The listing builds one solid part. Answer for the finished solid, in the listing's coordinates (mm). A direction names the side the tool comes from. Give positions to 0.01 mm unless a question says otherwise; leave off trailing zeros. Write each loop counter-clockwise with the first axis right and the second up, starting at its lowest first coordinate (ties: lowest second). Pieces come first, ordered by that corner, then holes.
```python
from build123d import *

# Parameters (mm, degrees)
SKETCH_1_R      = 1.6
EXTRUDE_1_DEPTH = 2.5
FILLET_1_R      = 2


with BuildPart() as part:
    # 草图1 → 凸台-拉伸1 (new body)
    with BuildSketch(Plane(origin=(0, 0, 0), x_dir=(-1, 0, 0), z_dir=(0, 1, 0))):
        Polygon((-27.5, 21.5), (27.5, 21.5), (33.5, 21.5), (33.5, -12.5), (27.5, -12.5), (27.5, -21.5), (-27.5, -21.5), align=None)
        with Locations(Location((-24.5, 9.5, 0), (0, 0, 90))):
            Circle(SKETCH_1_R, mode=Mode.SUBTRACT)
        with Locations(Location((-9.5, 9.5, 0), (0, 0, 90))):
            Circle(SKETCH_1_R, mode=Mode.SUBTRACT)
        with Locations(Location((-24.5, -6.5, 0), (0, 0, 90))):
            Circle(SKETCH_1_R, mode=Mode.SUBTRACT)
        with Locations(Location((-9.5, -6.5, 0), (0, 0, 90))):
            Circle(SKETCH_1_R, mode=Mode.SUBTRACT)
        with Locations(Location((4.5, -2.5, 0), (0, 0, 90))):
            Circle(SKETCH_1_R, mode=Mode.SUBTRACT)
        with Locations(Location((4.5, 11.5, 0), (0, 0, 90))):
            Circle(SKETCH_1_R, mode=Mode.SUBTRACT)
        with Locations(Location((24.5, 11.5, 0), (0, 0, 90))):
            Circle(SKETCH_1_R, mode=Mode.SUBTRACT)
        with Locations(Location((16.5, -14.5, 0), (0, 0, 90))):
            Circle(SKETCH_1_R, mode=Mode.SUBTRACT)
        with Locations(Location((4.5, -18, 0), (0, 0, 90))):
            Circle(SKETCH_1_R, mode=Mode.SUBTRACT)
    extrude(amount=EXTRUDE_1_DEPTH)

    # 圆角1
    fillet_1_edges = [part.edges().sort_by_distance(p)[0] for p in [
        (27.5, 1.25, 21.5),
        (-33.5, 1.25, 21.5),
        (-33.5, 1.25, -12.5),
        (-27.5, 1.25, -12.5),
        (-27.5, 1.25, -21.5),
        (27.5, 1.25, -21.5),
    ]]
    fillet(fillet_1_edges, radius=FILLET_1_R)


solid = part.part
```
Item 1: A cutting plane is placed at A-A, the plane z = -2.5. Give the vertices of the cut face in (x, y), plus the area to 4 significant figures.
Conclusion:
outline: (-33.5, 0) - (-6.1, 0) - (-6.1, 2.5) - (-33.5, 2.5) - close; (-2.9, 0) - (27.5, 0) - (27.5, 2.5) - (-2.9, 2.5) - close
area: 144.5 mm2
Item 2: A cutting plane is placed at D-D, the plane x = -4.5. Give the vertices of the cut face in (y, z), plus the area to 3 significant figures.
Conclusion:
outline: (0, -21.5) - (2.5, -21.5) - (2.5, -19.6) - (0, -19.6) - close; (0, -16.4) - (2.5, -16.4) - (2.5, -4.1) - (0, -4.1) - close; (0, -0.9) - (2.5, -0.9) - (2.5, 9.9) - (0, 9.9) - close; (0, 13.1) - (2.5, 13.1) - (2.5, 21.5) - (0, 21.5) - close
area: 83.5 mm2
Item 3: This flat-tipped pin is pushed along its axis until it touches: P1, Ø0.6, axis at x = -30.5, y = 1.5, coming from the -Z side. Where does it stop, or does it pass through?
Conclusion:
P1: stops at z = -12.5
Item 4: Which of the six approach directions +Z, -Z, +X, -X, +Y, -Y give full straight-line access (tool end or side, diameter ignored) to faces 1 (the face through (-15.42, 1.23, -15.68)), 2 (the face through (-31, 1, -12.5))?
Conclusion:
face 1: +Y, -Y
face 2: -Z, -X, +Y, -Y
Item 5: A cutting plane is placed at C-C, the plane y = 0.55. Count the separate pieces of the cut face and the enclosed holes in it, plus the area to 3 significant figures.
Conclusion:
separate pieces: 1
enclosed holes: 9
area: 2,490 mm2
Item 6: Determine the mould class of faces 3 (the face through (-3, 2.5, 0)), 4 (the face through (-33.5, 1, 5)), 5 (the face through (-24.43, 1.23, 9.9)), 6 (the face through (27.5, 1, 0)) for opening direction X: pulls with the +X half, pulls with the -X half, needs draft (parallel to the pull), parting line crosses it, or undercut.
Conclusion:
face 3: needs draft
face 4: pulls with the -X half
face 5: undercut
face 6: pulls with the +X half
Item 7: Consider probe 1 along X at (y, z) = (1.3, 11.5); probe 2 along X at (y, z) = (1.2, -6.5); probe 3 along X at (y, z) = (1.45, -14.5). Determine where each line is inside the solid, lowest interval first.
Conclusion:
probe 1: x = -33.5 to -26.1, -22.9 to -6.1, -2.9 to 27.5
probe 2: x = -33.5 to 7.9, 11.1 to 22.9, 26.1 to 27.5
probe 3: x = -27.5 to -18.1, -14.9 to 27.5
Item 8: A cutting plane is placed at B-B, the plane x = -24.5. Give the vertices of the cut face in (y, z).
Conclusion:
outline: (0, -21.5) - (2.5, -21.5) - (2.5, 9.9) - (0, 9.9) - close; (0, 13.1) - (2.5, 13.1) - (2.5, 21.5) - (0, 21.5) - close
